Can you work these out from the model? Positions are in its coordinate system, mm. Give positions to 0.01 mm unless a question says otherwise; leave off trailing zeros. Loops run counter-clockwise (first coordinate to the right, second up) from the corner with the lowest first, then second, coordinate; pieces in that order, holes last. Notation, with made-up numbers: (84.25, 29.5) - (130.25, 29.5) arc R16 ccw to (130.25, 53.5) - close; hole circle Ø3 at (-4.75, 33). An arc over 180 degrees is marked (long way). Answer as a JSON object with one key per item and string values. Group by question number.
Item 1: Will this pin go through, and if not, where does the flat tip stop? pin 1 (10 mm diameter, centred on x = 13.5, y = -9, fed in from -Z).
Item 2: Please list where these lines run through material, in increasing order: L1, parallel to Y at x = 0, z = 1.8 (3 decimals); L2, parallel to X at y = 14.5, z = 0.1; L3, parallel to X at y = -13, z = 0.6.
Item 3: Suppose I cut it at A-A on x = 0. Write out the boundary of the cut face in (y, z) (3 decimals).
Item 4: Suppose I cut it at B-B on x = 46.99. Write out the boundary of the cut face in (y, z) (1 decimal), and give its area (3 significant figures).
Item 5: Thinking about a two-plate mould opening in Y: for faces 1 (the cylindrical face through (-53.886, -20.191, 1.03)), 2 (the cylindrical face through (45.34, 14.36, 1.25)), 3 (the cylindrical face through (53.846, 20.231, 1.03)), 4 (the cylindrical face through (45.68, -15.29, 1.25)), which applies, pulls with the +Y half, pulls with the -Y half, needs draft (parallel to the pull), parting line crosses it, or undercut?
from build123d import *

# Parameters (mm, degrees)
SKETCH1_W               = 109.22
SKETCH1_H               = 41.91
BOSS_EXTRUDE1_DEPTH     = 2.54
CUT_EXTRUDE2_DEPTH      = 59.547550974
CUT_EXTRUDE2_DEPTH_BACK = 59.547550974
SKETCH4_R               = 1.651
FILLET1_R               = 2.54
SKETCH14_R              = 1.651
CUT_EXTRUDE8_DEPTH      = 59.547550974
CHAMFER2_SIZE           = 0.508


with BuildPart() as part:
    # Sketch1 → Boss-Extrude1 (new body)
    with BuildSketch(Plane.XY):
        Rectangle(SKETCH1_W, SKETCH1_H)
    extrude(amount=BOSS_EXTRUDE1_DEPTH)

    # Sketch4 → Cut-Extrude2 (cut, two sides: drawn at the far end of the back side and taken through both)
    with BuildSketch(Plane.XY.offset(2.54).offset(-CUT_EXTRUDE2_DEPTH_BACK)):
        with Locations((-46.99, 14.2875)):
            Circle(SKETCH4_R)
        with Locations((-46.99, -14.2875)):
            Circle(SKETCH4_R)
        with Locations((46.99, -14.2875)):
            Circle(SKETCH4_R)
        with Locations((46.99, 14.2875)):
            Circle(SKETCH4_R)
    extrude(amount=CUT_EXTRUDE2_DEPTH + CUT_EXTRUDE2_DEPTH_BACK, mode=Mode.SUBTRACT)

    # Fillet1
    fillet1_edges = [part.edges().sort_by_distance(p)[0] for p in [
        (-54.61, 20.955, 1.27),
        (54.61, 20.955, 1.27),
        (54.61, -20.955, 1.27),
        (-54.61, -20.955, 1.27),
    ]]
    fillet(fillet1_edges, radius=FILLET1_R)

    # Sketch14 → Cut-Extrude8 (cut, through all)
    with BuildSketch(Plane.XY.offset(2.54)):
        with Locations((0, 17.145)):
            Circle(SKETCH14_R)
    extrude(amount=-CUT_EXTRUDE8_DEPTH, mode=Mode.SUBTRACT)

    # Chamfer2
    chamfer2_edges = [part.edges().sort_by_distance(p)[0] for p in [
        (0, 20.955, 2.54),
        (54.61, 0, 2.54),
        (-54.61, 0, 2.54),
        (0, -20.955, 2.54),
        (-53.866051224, 20.211051224, 2.54),
        (-53.866051224, -20.211051224, 2.54),
        (53.866051224, -20.211051224, 2.54),
        (53.866051224, 20.211051224, 2.54),
    ]]
    chamfer(chamfer2_edges, length=CHAMFER2_SIZE)


solid = part.part
Worked out:
{
 "1": {"pin 1": "stops at z = 0"},
 "2": {"L1": "y = -20.955 to 15.494, 18.796 to 20.955", "L2": "x = -54.61 to -48.63, -45.35 to 45.35, 48.63 to 54.61", "L3": "x = -54.61 to -48.02, -45.96 to 45.96, 48.02 to 54.61"},
 "3": {"outline": "(-20.955, 0) - (15.494, 0) - (15.494, 2.54) - (-20.447, 2.54) - (-20.955, 2.032) - close; (18.796, 0) - (20.955, 0) - (20.955, 2.032) - (20.447, 2.54) - (18.796, 2.54) - close"},
 "4": {"outline": "(-21, 0) - (-15.9, 0) - (-15.9, 2.5) - (-20.4, 2.5) - (-21, 2) - close; (-12.6, 0) - (12.6, 0) - (12.6, 2.5) - (-12.6, 2.5) - close; (15.9, 0) - (21, 0) - (21, 2) - (20.4, 2.5) - (15.9, 2.5) - close", "area": "89.4 mm2"},
 "5": {"face 1": "pulls with the -Y half", "face 2": "undercut", "face 3": "pulls with the +Y half", "face 4": "undercut"}
}
